Here's the drawing with two shaded views (mm, measured from the low corner). I have some questions. A direction names the side the tool comes from. Coordinates: 2 decimals unless noted, no trailing zeros. Write each loop counter-clockwise with the first axis right and the second up, starting at its lowest first coordinate (ties: lowest second). Pieces come first, ordered by that corner, then holes.
Item 1: I'm going to push flat-ended pins straight in: pin 1 Ø17.5 at (x, y) = (30.5, 20.5) entering from -Z; pin 2 Ø6 at (y, z) = (20.5, 6.5) entering from -X; pin 3 Ø4.5 at (y, z) = (41.86, 5) entering from +X; pin 4 Ø24 at (x, y) = (20.5, 21) entering from +Z. Where does each tip first touch, or does it pass through?
Item 2: If we section it at A-A (y = 9): Please give me the cut outline in (x, z), then the cut area to 3 significant figures.
Item 3: If I drill on line 1 (Z direction, x = 23.5, y = 24); line 2 (Z direction, x = 3, y = 41) (1 decimal); line 3 (X direction, y = 24.5, z = 26.5), over which ranges is the centre line in solid material (lowest first)?
Item 4: If we section it at C-C (z = 17): Please give me the cut outline in (x, y).
Item 5: For the marked faces 1, 2 and 3, which set-ups out of +Z, -Z, +X, -X, +Y, -Y let a thin tool reach every point of the face, with its end or its side?
Item 6: If we section it at D-D (y = 36): Please give me the cut outline in (x, z).
Item 7: If we section it at B-B (z = 5): Count the separate pieces of the cut face and the enclosed holes in it, then the cut area to 3 significant figures.
Item 8: We'd pull the mould along Z, two halves only. Please class the marked faces 4, 5, 6 and 7: +Z half, -Z half, draft (parallel to the pull), parting line (faces both ways), or undercut.
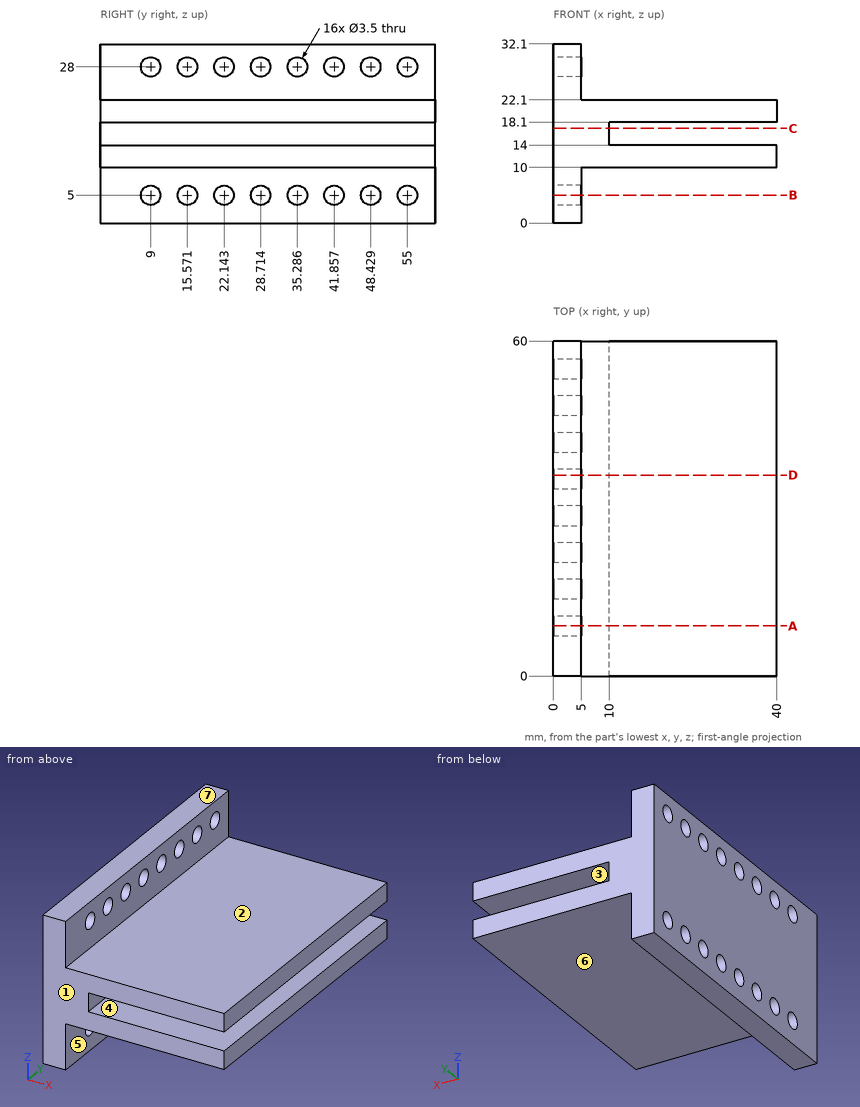
Answer list:
1. pin 1: stops at z = 10
1. pin 2: stops at x = 0
1. pin 3: stops at x = 5
1. pin 4: stops at z = 22.1
2. outline: (0, 0) - (5, 0) - (5, 3.25) - (0, 3.25) - close; (0, 6.75) - (5, 6.75) - (5, 10) - (40, 10) - (40, 14) - (10, 14) - (10, 18.1) - (40, 18.1) - (40, 22.1) - (5, 22.1) - (5, 26.25) - (0, 26.25) - close; (0, 29.75) - (5, 29.75) - (5, 32.1) - (0, 32.1) - close
2. area: 426 mm2
3. line 1: z = 10 to 14, 18.1 to 22.1
3. line 2: z = 0 to 3.5, 6.5 to 26.5, 29.5 to 32.1
3. line 3: x = 0 to 5
4. outline: (0, 0) - (10, 0) - (10, 60) - (0, 60) - close
5. face 1: +Z, -Z, +X, -X, -Y
5. face 2: +Z, +X, +Y, -Y
5. face 3: +X, +Y, -Y
6. outline: (0, 0) - (5, 0) - (5, 3.4) - (0, 3.4) - close; (0, 6.6) - (5, 6.6) - (5, 10) - (40, 10) - (40, 14) - (10, 14) - (10, 18.1) - (40, 18.1) - (40, 22.1) - (5, 22.1) - (5, 26.4) - (0, 26.4) - close; (0, 29.6) - (5, 29.6) - (5, 32.1) - (0, 32.1) - close
7. separate pieces: 9
7. enclosed holes: 0
7. area: 160 mm2
8. face 4: undercut
8. face 5: draft
8. face 6: -Z half
8. face 7: +Z half
